Can you work these out from the drawing? Everything is in mm from the part's minimum corner. A direction names the side the tool comes from. Coordinates: 2 decimals unless noted, no trailing zeros. Order: outer loops, then holes, each group sorted by start corner. A loop starts at its lowest first (then second) coordinate and runs counter-clockwise, first axis right, second up. Notation, with made-up numbers: (-25.75, 43.5) -> (-21.75, 43.5) arc R18 ccw to (-21.75, 62.5) -> close; hole circle Ø11 at (-24.5, -39.75). An arc over 180 degrees is marked (long way). Answer in a Markdown table with one row per item.
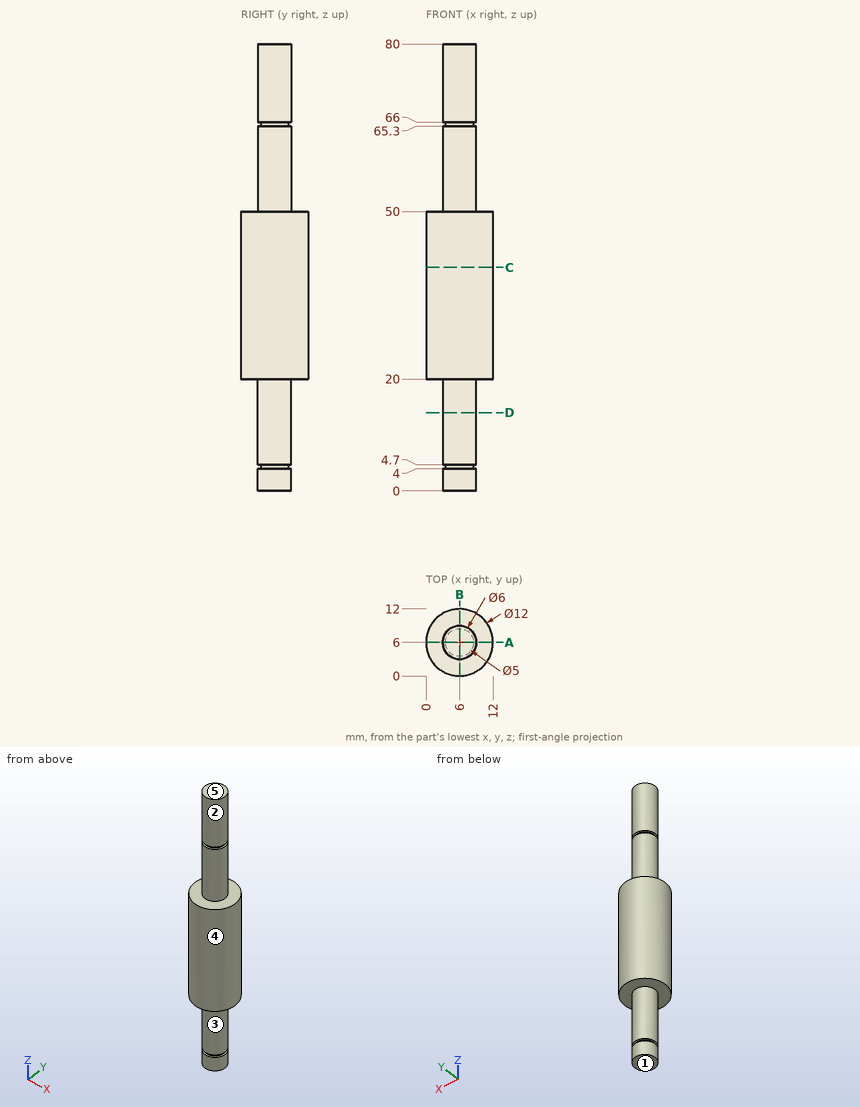
(1) Will these pins go through, and if not, where does the flat tip stop? pin 1 Ø3 at (x, y) = (7, 5) entering from -Z; pin 2 Ø1 at (y, z) = (3.5, 59.5) entering from -X.
Response values:
| item | result |
|---|---|
| pin 1 | z = 0 |
| pin 2 | x = 3.76 |
(2) Suppose I cut it at D-D (z = 14). Please give me the cut outline in (x, y).
Response values:
| item | result |
|---|---|
| outline | circle Ø6 at (6, 6) |
(3) We'd pull the mould along Y, two halves only. Please class the marked faces 4 and 5: +Y half, -Y half, draft (parallel to the pull), parting line (faces both ways), or undercut.
Response values:
| item | result |
|---|---|
| face 4 | parting line |
| face 5 | draft |
(4) I need wall thicknesses on line 1 (Z direction, x = 8.75, y = 6.5); line 2 (X direction, y = 5.75, z = 10); line 3 (Y direction, x = 6, z = 19.5). Which ranges of each line are inside material? Lowest first, please. Write a range as [from, to].
Response values:
| item | result |
|---|---|
| line 1 | [0, 4], [4.7, 65.3], [66, 80] |
| line 2 | [3.01, 8.99] |
| line 3 | [3, 9] |
(5) Suppose I cut it at C-C (z = 40). Please give me the cut outline in (x, y), and give its area (3 significant figures).
Response values:
| item | result |
|---|---|
| outline | circle Ø12 at (6, 6) |
| area | 113 mm2 |
(6) On a 3-axis mill with a long thin cutter (end or side, diameter ignored), from which of +Z, -Z, +X, -X, +Y, -Y can I reach the whole of each face in a straight line? I mean the marked faces 1, 2 and 3. Say none if no direction works.
Response values:
| item | result |
|---|---|
| face 1 | -Z, +X, -X, +Y, -Y |
| face 2 | +Z |
| face 3 | -Z |
(7) Suppose I cut it at A-A (y = 6). Please give me the cut outline in (x, z), and give its area (3 significant figures).
Response values:
| item | result |
|---|---|
| outline | (0, 20) -> (3, 20) -> (3, 4.7) -> (3.5, 4.7) -> (3.5, 4) -> (3, 4) -> (3, 0) -> (9, 0) -> (9, 4) -> (8.5, 4) -> (8.5, 4.7) -> (9, 4.7) -> (9, 20) -> (12, 20) -> (12, 50) -> (9, 50) -> (9, 65.3) -> (8.5, 65.3) -> (8.5, 66) -> (9, 66) -> (9, 80) -> (3, 80) -> (3, 66) -> (3.5, 66) -> (3.5, 65.3) -> (3, 65.3) -> (3, 50) -> (0, 50) -> close |
| area | 659 mm2 |
